Autodesk Inventor part; units mm, degrees
ref_plane "YZ Plane" through (0, 0, 0) normal (1, 0, 0) x (0, 1, 0)
ref_plane "XZ Plane" through (0, 0, 0) normal (0, 1, 0) x (-1, 0, 0)
ref_plane "XY Plane" through (0, 0, 0) normal (0, 0, 1) x (1, 0, 0)
sketch "Sketch1" plane through (0, 0, 0) normal (0, 0, 1) x (1, 0, 0)
  line L0 (0, 0) -> (25.4, 0)
  line L1 (25.4, 0) -> (25.4, 25.4)
  line L2 (25.4, 25.4) -> (0, 25.4)
  line L3 (0, 25.4) -> (0, 0)
  dimension "d0" = 25.4
  dimension "d1" = 25.4
extrude "Extrusion1" add sketch "Sketch1" along normal blind 546.1
shell "Shell1" thickness 2.54 removed faces 2 at (8.4667, 16.9333, 0) at (8.4667, 16.9333, 546.1)
sketch "Sketch2" plane through (0, 25.4, 0) normal (0, 1, 0) x (1, 0, 0)
  line L0 (25.4, 0) -> (0, 0)
  line L1 (0, 0) -> (0, -546.1)
  point P0 (12.7, -12.7)
  point P1 (12.7, -38.1)
  point P2 (12.7, -63.5)
  point P3 (12.7, -88.9)
  point P4 (12.7, -114.3)
  point P5 (12.7, -139.7)
  point P6 (12.7, -165.1)
  point P7 (12.7, -190.5)
  point P8 (12.7, -215.9)
  point P9 (12.7, -241.3)
  point P10 (12.7, -266.7)
  point P11 (12.7, -292.1)
  point P12 (12.7, -317.5)
  point P13 (12.7, -342.9)
  point P14 (12.7, -368.3)
  point P15 (12.7, -393.7)
  point P16 (12.7, -419.1)
  point P17 (12.7, -444.5)
  point P18 (12.7, -469.9)
  point P19 (12.7, -495.3)
  point P20 (12.7, -520.7)
  point P21 (12.7, -546.1)
  point P22 (12.7, -571.5)
  point P23 (12.7, -596.9)
  point P24 (12.7, -622.3)
  point P25 (12.7, -647.7)
  point P26 (12.7, -673.1)
  point P27 (12.7, -698.5)
  point P28 (12.7, -723.9)
  point P29 (12.7, -749.3)
  point P30 (12.7, -774.7)
  point P31 (12.7, -800.1)
  point P32 (12.7, -825.5)
  point P33 (12.7, -850.9)
  point P34 (12.7, -876.3)
  point P35 (12.7, -901.7)
  point P36 (12.7, -927.1)
  dimension "d5" = 12.7
  dimension "d6" = 12.7
  dimension "d9" = 25.4
hole "Hole1" at (12.7, 25.4, 12.7) at (12.7, 25.4, 38.1) at (12.7, 25.4, 63.5) at (12.7, 25.4, 88.9) at (12.7, 25.4, 114.3) at (12.7, 25.4, 139.7) at (12.7, 25.4, 165.1) at (12.7, 25.4, 190.5) at (12.7, 25.4, 215.9) at (12.7, 25.4, 241.3) at (12.7, 25.4, 266.7) at (12.7, 25.4, 292.1) at (12.7, 25.4, 317.5) at (12.7, 25.4, 342.9) at (12.7, 25.4, 368.3) at (12.7, 25.4, 393.7) at (12.7, 25.4, 419.1) at (12.7, 25.4, 444.5) at (12.7, 25.4, 469.9) at (12.7, 25.4, 495.3) at (12.7, 25.4, 520.7) at (12.7, 25.4, 546.1) at (12.7, 25.4, 571.5) at (12.7, 25.4, 596.9) at (12.7, 25.4, 622.3) at (12.7, 25.4, 647.7) at (12.7, 25.4, 673.1) at (12.7, 25.4, 698.5) at (12.7, 25.4, 723.9) at (12.7, 25.4, 749.3) at (12.7, 25.4, 774.7) at (12.7, 25.4, 800.1) at (12.7, 25.4, 825.5) at (12.7, 25.4, 850.9) at (12.7, 25.4, 876.3) at (12.7, 25.4, 901.7) direction (0, -1, 0) diameter 2.54 depth 50.8 tip angle 118
properties part number "cross bar 2" material "Aluminum 6061"
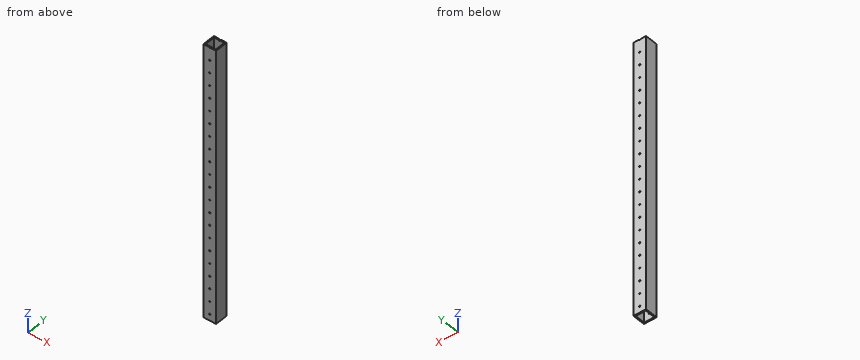
The model under review builds one solid part; all positions refer to its coordinate system, in mm. Round coordinates to 2 decimals unless told otherwise and drop trailing zeros. Order: outer loops, then holes, each group sorted by start corner. A loop starts at its lowest first (then second) coordinate and runs counter-clockwise, first axis right, second up.
(1) Wall thickness on L1, parallel to Y at x = 13.5, z = 185; L2, parallel to X at y = 1.2, z = 292.1: over which ranges is each line inside the solid? List them lowest first.
Working result:
L1: y = 0 to 2.54, 22.86 to 25.4
L2: x = 0 to 11.43, 13.97 to 25.4
(2) For P1, Ø1.5, axis at x = 21.5, y = 19, coming from the -Z side, flat-tipped, find the tip position at first contact; note if it passes through.
Working result:
P1: passes through
(3) Take a section at A-A, the plane y = 7. State the section outline as (x, z) points, plus the area to 3 significant figures.
Working result:
outline: (0, 0) - (2.54, 0) - (2.54, 546.1) - (0, 546.1) - close; (22.86, 0) - (25.4, 0) - (25.4, 546.1) - (22.86, 546.1) - close
area: 2,770 mm2
(4) Take a section at B-B, the plane z = 57. State the section outline as (x, y) points, plus the area to 3 significant figures.
Working result:
outline: (0, 0) - (25.4, 0) - (25.4, 25.4) - (0, 25.4) - close; hole (2.54, 2.54) - (22.86, 2.54) - (22.86, 22.86) - (2.54, 22.86) - close
area: 232 mm2
